```python
from build123d import *

# Parameters (mm, degrees)
SKETCH1_W           = 72
SKETCH1_H           = 83
BOSS_EXTRUDE1_DEPTH = 18
CAVITY2_START       = -80.5
CAVITY2_DEPTH       = 34
CAVITY2_START_2     = -48.5
CAVITY2_2_DEPTH     = 46
CAVITY2_3_DEPTH     = 5
CAVITY2_START_3     = -51.5
CAVITY2_4_DEPTH     = 5
CAVITY2_START_4     = -4.5
CAVITY2_5_OUTLINE_W = 37
CAVITY2_5_OUTLINE_H = 5
CAVITY2_5_DEPTH     = 2
CAVITY2_6_DEPTH     = 2
CAVITY2_7_DEPTH     = 2


# Read off the part's stored shape, not the designer's step: Cavity2
with BuildPart() as part:
    # Sketch1 → Boss-Extrude1 (new body)
    with BuildSketch(Plane(origin=(0, 0, 0), x_dir=(1, 0, 0), z_dir=(0, 1, 0))):
        with Locations((36, 41.5)):
            Rectangle(SKETCH1_W, SKETCH1_H)
    extrude(amount=BOSS_EXTRUDE1_DEPTH)

    # Cavity2 outline → Cavity2 (cut)
    with BuildSketch(Plane.XY.offset(CAVITY2_START)):
        Polygon((55.404610688, 2), (55.404610688, 12.86969785), (69.5, 18), (47.804610688, 18), (47.804610688, 2), align=None)
        Polygon((24.804610688, 18), (3.109221376, 18), (17.204610688, 12.86969785), (17.204610688, 2), (24.804610688, 2), align=None)
    extrude(amount=CAVITY2_DEPTH, mode=Mode.SUBTRACT)

    # Cavity2 2 outline → Cavity2 2 (cut)
    with BuildSketch(Plane.XY.offset(CAVITY2_START_2)):
        Polygon((55.404610688, 11), (57.404610688, 11), (57.404610688, 18), (8.404610688, 18), (8.404610688, 11), (10.404610688, 11), (10.404610688, 16), (16.404610688, 16), (16.404610688, 11), (18.404610688, 11), (18.404610688, 16), (55.404610688, 16), align=None)
    extrude(amount=CAVITY2_2_DEPTH, mode=Mode.SUBTRACT)

    # Cavity2 3 outline → Cavity2 3 (cut)
    with BuildSketch(Plane.XY.offset(CAVITY2_START)):
        Polygon((47.804610688, 2), (47.804610688, 18), (24.804610688, 18), (24.804610688, 2), (27.904610688, 2), (27.904610688, 16), (31.904610688, 16), (31.904610688, 2), align=None)
    extrude(amount=CAVITY2_3_DEPTH, mode=Mode.SUBTRACT)

    # Cavity2 4 outline → Cavity2 4 (cut)
    with BuildSketch(Plane.XY.offset(CAVITY2_START_3)):
        Polygon((47.804610688, 2), (47.804610688, 18), (24.804610688, 18), (24.804610688, 2), (40.704610688, 2), (40.704610688, 16), (44.704610688, 16), (44.704610688, 2), align=None)
    extrude(amount=CAVITY2_4_DEPTH, mode=Mode.SUBTRACT)

    # Cavity2 5 outline → Cavity2 5 (cut)
    with BuildSketch(Plane.XY.offset(CAVITY2_START_4)):
        with Locations((36.904610688, 13.5)):
            Rectangle(CAVITY2_5_OUTLINE_W, CAVITY2_5_OUTLINE_H)
    extrude(amount=CAVITY2_5_DEPTH, mode=Mode.SUBTRACT)

    # Cavity2 6 outline → Cavity2 6 (cut)
    with BuildSketch(Plane.XY.offset(CAVITY2_START)):
        Polygon((55.404610688, 7.548808988), (69.5, 12.679111138), (69.5, 18), (55.404610688, 12.86969785), align=None)
        Polygon((3.109221376, 18), (3.109221376, 12.679111138), (17.204610688, 7.548808988), (17.204610688, 12.86969785), align=None)
    extrude(amount=CAVITY2_6_DEPTH, mode=Mode.SUBTRACT)

    # Cavity2 7 outline → Cavity2 7 (cut)
    with BuildSketch(Plane.XY.offset(CAVITY2_START_2)):
        Polygon((55.404610688, 7.548808988), (69.5, 12.679111138), (69.5, 18), (57.404610688, 13.597638319), (57.404610688, 11), (55.404610688, 11), align=None)
        Polygon((8.404610688, 11), (8.404610688, 16.072635912), (3.109221376, 18), (3.109221376, 12.679111138), (17.204610688, 7.548808988), (17.204610688, 11), (16.404610688, 11), (16.404610688, 13.160874037), (10.404610688, 15.344695443), (10.404610688, 11), align=None)
    extrude(amount=CAVITY2_7_DEPTH, mode=Mode.SUBTRACT)


solid = part.part
```
Read the model definition and answer for the solid it produces. Units are mm, in the model's axes. A direction names the side the tool comes from. Coordinates: 2 decimals unless noted, no trailing zeros. Write each loop counter-clockwise with the first axis right and the second up, starting at its lowest first coordinate (ties: lowest second). Pieces come first, ordered by that corner, then holes. Notation, with made-up numbers: (14, -31) -> (23, -31) arc R4 cw to (23, -24) -> close; hole circle Ø7 at (-22, 20). An arc over 180 degrees is marked (long way). Answer as a JSON object with one key per item and string values.
Q1. Determine the mould class of faces 1 (the flat face through (38, 15, -2.5)), 2 (the flat face through (24, 2, -60)), 3 (the flat face through (35, 9, 0)), 4 (the flat face through (35, 9, -83)) for opening direction Z: pulls with the +Z half, pulls with the -Z half, needs draft (parallel to the pull), parting line crosses it, or undercut.
The answers:
{"face 1": "undercut", "face 2": "undercut", "face 3": "pulls with the +Z half", "face 4": "pulls with the -Z half"}
Q2. The part is cut by section D-D on z = -34. Give the vertices of the cut face in (x, y), then the cut area to 3 significant figures.
The answers:
{"outline": "(0, 0) -> (72, 0) -> (72, 18) -> (57.4, 18) -> (57.4, 11) -> (55.4, 11) -> (55.4, 16) -> (18.4, 16) -> (18.4, 11) -> (16.4, 11) -> (16.4, 16) -> (10.4, 16) -> (10.4, 11) -> (8.4, 11) -> (8.4, 18) -> (0, 18) -> close", "area": "1,170 mm2"}
Q3. The part is cut by section C-C on x = 26. Give the vertices of the cut face in (y, z), then the cut area to 3 significant figures.
The answers:
{"outline": "(0, -83) -> (18, -83) -> (18, -80.5) -> (2, -80.5) -> (2, -75.5) -> (18, -75.5) -> (18, -51.5) -> (2, -51.5) -> (2, -46.5) -> (16, -46.5) -> (16, -4.5) -> (11, -4.5) -> (11, -2.5) -> (18, -2.5) -> (18, 0) -> (0, 0) -> close", "area": "1,240 mm2"}
Q4. A flat-ended cylindrical pin translates along its axis: pin 1 Ø6.5 at (x, z) = (13.5, -24) entering from +Y. Find the tip coordinate at first contact, or state that the pin passes through.
The answers:
{"pin 1": "stops at y = 16"}
Q5. The part is cut by section A-A on z = -77. Give the vertices of the cut face in (x, y), then the cut area to 3 significant figures.
The answers:
{"outline": "(0, 0) -> (72, 0) -> (72, 18) -> (69.5, 18) -> (55.4, 12.87) -> (55.4, 2) -> (31.9, 2) -> (31.9, 16) -> (27.9, 16) -> (27.9, 2) -> (17.2, 2) -> (17.2, 12.87) -> (3.11, 18) -> (0, 18) -> close", "area": "668 mm2"}
Q6. A tool of negligible diameter and unlimited length cuts with its end or side. For faces 5 (the flat face through (0, 9, -41)), 6 (the flat face through (9, 11, -25)), from which of +Z, -Z, +X, -X, +Y, -Y can it reach the whole face along a straight path? Write none if from no direction.
The answers:
{"face 5": "+Z, -Z, -X, +Y, -Y", "face 6": "+Y"}
Q7. The part is cut by section B-B on y = 9. Give the vertices of the cut face in (x, z), then the cut area to 3 significant figures.
The answers:
{"outline": "(0, -83) -> (72, -83) -> (72, 0) -> (0, 0) -> close; hole (13.22, -80.5) -> (27.9, -80.5) -> (27.9, -75.5) -> (24.8, -75.5) -> (24.8, -51.5) -> (40.7, -51.5) -> (40.7, -46.5) -> (13.22, -46.5) -> (13.22, -48.5) -> (17.2, -48.5) -> (17.2, -78.5) -> (13.22, -78.5) -> close; hole (31.9, -80.5) -> (59.39, -80.5) -> (59.39, -78.5) -> (55.4, -78.5) -> (55.4, -48.5) -> (59.39, -48.5) -> (59.39, -46.5) -> (44.7, -46.5) -> (44.7, -51.5) -> (47.8, -51.5) -> (47.8, -75.5) -> (31.9, -75.5) -> close", "area": "5,240 mm2"}
Q8. Consider line 1 (X direction, y = 5, z = -65.5); line 2 (X direction, y = 14.5, z = -13.5); line 3 (X direction, y = 3.25, z = -79.5). Determine where each line is inside the solid, lowest interval first. Write a range as [from, to].
The answers:
{"line 1": "x = [0, 17.2], [24.8, 47.8], [55.4, 72]", "line 2": "x = [0, 8.4], [10.4, 16.4], [18.4, 55.4], [57.4, 72]", "line 3": "x = [0, 17.2], [27.9, 31.9], [55.4, 72]"}
